The listing builds one solid part. Answer for the finished solid, in the listing's coordinates (mm). Give positions to 0.01 mm unless a question says otherwise; leave off trailing zeros. Order: outer loops, then holes, each group sorted by start corner. A loop starts at its lowest first (then second) coordinate and runs counter-clockwise, first axis right, second up. Notation, with made-up numbers: (-19.5, -39.5) - (5.5, -39.5) arc R25 cw to (5.5, -13.5) - close; hole circle Ø11 at (-38.75, 73). An arc over 180 degrees is marked (long way). Answer in a Markdown table with one row per item. Add a question column.
```python
from build123d import *

# Parameters (mm, degrees)
SKETCH1_R           = 13
BOSS_EXTRUDE1_DEPTH = 3
SKETCH3_R           = 2.25
CUT_EXTRUDE1_DEPTH  = 3
SKETCH2_R           = 1.75
CUT_EXTRUDE2_DEPTH  = 3


with BuildPart() as part:
    # Sketch1 → Boss-Extrude1 (new body)
    with BuildSketch(Plane(origin=(0, 0, 0), x_dir=(1, 0, 0), z_dir=(0, 1, 0))):
        with Locations(Location((0, 0, 0), (0, 0, 270))):
            Circle(SKETCH1_R)
    extrude(amount=BOSS_EXTRUDE1_DEPTH)

    # Sketch3 → Cut-Extrude1 (cut)
    with BuildSketch(Plane(origin=(0, 3, 0), x_dir=(1, 0, 0), z_dir=(0, 1, 0))):
        with Locations(Location((0, 0, 0), (0, 0, 270))):
            Circle(SKETCH3_R)
    extrude(amount=-CUT_EXTRUDE1_DEPTH, mode=Mode.SUBTRACT)

    # Sketch2 → Cut-Extrude2 (cut)
    with BuildSketch(Plane(origin=(0, 3, 0), x_dir=(1, 0, 0), z_dir=(0, 1, 0))):
        with Locations(Location((9, 0, 0), (0, 0, 270))):
            Circle(SKETCH2_R)
    cut_extrude2 = extrude(amount=-CUT_EXTRUDE2_DEPTH, mode=Mode.SUBTRACT)

    # Mirror1: Cut-Extrude2 across plane
    add(cut_extrude2.mirror(Plane(origin=(0, 0, 0), x_dir=(0, 0, 1), z_dir=(1, 0, 0))), mode=Mode.SUBTRACT)


solid = part.part
```
(1) The mould has two halves that part along Z. Classify faces 1 (the face through (-10.735, 1.521, -0.228)), 2 (the face through (-7.91, 1.479, -10.316)), 3 (the face through (0, 0, 3)): +Z half, -Z half, draft (parallel to the pull), parting line (faces both ways), or undercut.
(2) Find section C-C, the plane y = 2.7. Write down the section's boundary in (x, z).
(3) Straight lines are drawn through the part: line 1 (X direction, y = 2.15, z = 0); line 2 (Z direction, x = -9, y = 1.1); line 3 (Z direction, x = 9.75, y = 1.25). For each, find the intervals that lie inside material, in ascending order.
(4) Find section B-B, the plane z = 0. Write down the section's boundary in (x, y).
(5) Find section A-A, the plane x = 0. Write down the section's boundary in (y, z).
(6) Each of these flat-tipped pins is pushed along its axis until it touches: P1, Ø1, axis at x = 1.5, y = 1.5, coming from the -Z side; P2, Ø1, axis at x = 1, y = 1.5, coming from the +Z side; P3, Ø1.5, axis at x = -4, y = 2, coming from the -Z side; P4, Ø2, axis at x = -9, z = 0, coming from the +Y side. Where does it stop, or does it pass through?
(7) Find section D-D, the plane x = 9. Write down the section's boundary in (y, z).
Answer key:
| question | item | result |
|---|---|---|
| 1 | face 1 | undercut |
| 1 | face 2 | parting line |
| 1 | face 3 | draft |
| 2 | outline | circle Ø26 at (0, 0); hole circle Ø3.5 at (-9, 0); hole circle Ø4.5 at (0, 0); hole circle Ø3.5 at (9, 0) |
| 3 | line 1 | -13 to -10.75, -7.25 to -2.25, 2.25 to 7.25, 10.75 to 13 |
| 3 | line 2 | -9.38 to -1.75, 1.75 to 9.38 |
| 3 | line 3 | -8.6 to -1.58, 1.58 to 8.6 |
| 4 | outline | (-13, 0) - (-10.75, 0) - (-10.75, 3) - (-13, 3) - close; (-7.25, 0) - (-2.25, 0) - (-2.25, 3) - (-7.25, 3) - close; (2.25, 0) - (7.25, 0) - (7.25, 3) - (2.25, 3) - close; (10.75, 0) - (13, 0) - (13, 3) - (10.75, 3) - close |
| 5 | outline | (0, -13) - (3, -13) - (3, -2.25) - (0, -2.25) - close; (0, 2.25) - (3, 2.25) - (3, 13) - (0, 13) - close |
| 6 | P1 | z = -12.96 |
| 6 | P2 | z = 12.99 |
| 6 | P3 | z = -12.59 |
| 6 | P4 | through |
| 7 | outline | (0, -9.38) - (3, -9.38) - (3, -1.75) - (0, -1.75) - close; (0, 1.75) - (3, 1.75) - (3, 9.38) - (0, 9.38) - close |
